Autodesk Inventor part; units mm, degrees
ref_plane "Work Plane1" through (-12, 0, -50) normal (0, -1, 0) x (1, 0, 0)
ref_plane "YZ Plane" through (0, 0, 0) normal (1, 0, 0) x (0, 1, 0)
ref_plane "XZ Plane" through (0, 0, 0) normal (0, 1, 0) x (-1, 0, 0)
sketch "Sketch1" plane through (0, 0, 0) normal (0, 1, 0) x (-1, 0, 0)
  line L0 (12, 50) -> (-12, 50)
  line L1 (-12, 50) -> (-12, -50)
  line L2 (-12, -50) -> (12, -50)
  line L3 (12, -50) -> (12, 50)
  line L4 (12, 50) -> (-12, -50) construction
  line L5 (-12, 50) -> (12, -50) construction
  point P0 (0, 0)
  dimension "d0" = 24
  dimension "d1" = 100
  dimension "d135" = 50
extrude "Extrusion1" add sketch "Sketch1" along normal blind 5
sketch "Sketch3" plane through (0, 5, 0) normal (0, 1, 0) x (1, 0, 0)
  line L0 (-0.2475, -27) -> (0.2525, -27)
  line L1 (0.2525, -27) -> (0.2525, -49)
  line L2 (0.2525, -49) -> (-0.2475, -49)
  line L3 (-0.2475, -49) -> (-0.2475, -27)
  line L4 (12, -50) -> (12, 50)
  line L5 (-12, 50) -> (-12, -50)
  line L6 (-12, -50) -> (12, -50)
  point P0 (0, 0)
  dimension "d24" = 0.5
  dimension "d25" = 11.7475
  dimension "d26" = 22
  dimension "d97" = 11.7525
  dimension "d113" = 1
extrude "Extrusion3" add sketch "Sketch3" along normal blind 30
sketch "Sketch4" plane through (0, 5, 0) normal (0, 1, 0) x (1, 0, 0)
  line L0 (-9.1, -27) -> (9.1, -27)
  line L1 (9.1, -27) -> (9.1, -28)
  line L2 (9.1, -28) -> (-9.1, -28)
  line L3 (-9.1, -28) -> (-9.1, -27)
  line L4 (12, -50) -> (12, 50)
  line L5 (-12, 50) -> (-12, -50)
  line L6 (-12, -50) -> (12, -50)
  point P0 (0, 0)
  dimension "d29" = 1
  dimension "d30" = 2.9
  dimension "d31" = 2.9
  dimension "d114" = 22
extrude "Extrusion4" add sketch "Sketch4" along normal blind 30
sketch "Sketch7" plane through (0, 5, 0) normal (0, 1, 0) x (1, 0, 0)
  line L0 (9.1, -27) -> (8.1, -27)
  line L1 (8.1, -27) -> (8.1, -49)
  line L2 (8.1, -49) -> (9.1, -49)
  line L3 (9.1, -49) -> (9.1, -27)
  line L4 (12, -50) -> (12, 50)
  point P0 (0, 0)
  dimension "d46" = 22
  dimension "d47" = 2.9
  dimension "d48" = 1
extrude "Extrusion7" add sketch "Sketch7" along normal blind 30
sketch "Sketch8" plane through (0, 5, 0) normal (0, 1, 0) x (1, 0, 0)
  line L0 (-9.1, -28) -> (-8.1, -28)
  line L1 (-8.1, -28) -> (-8.1, -49)
  line L2 (-8.1, -49) -> (-9.1, -49)
  line L3 (-9.1, -49) -> (-9.1, -28)
  line L4 (-12, 50) -> (-12, -50)
  point P0 (0, 0)
  dimension "d51" = 21
  dimension "d52" = 2.9
  dimension "d53" = 1
extrude "Extrusion8" add sketch "Sketch8" along normal blind 30
sketch "Sketch9" plane through (0, 5, 0) normal (0, 1, 0) x (1, 0, 0)
  line L0 (-8.3501, -48) -> (-0.2475, -48)
  line L1 (-0.2475, -48) -> (-0.2475, -49)
  line L2 (-0.2475, -49) -> (-8.3501, -49)
  line L3 (-8.3501, -49) -> (-8.3501, -48)
  line L4 (-0.2475, -49) -> (-0.2475, -27)
  line L5 (-12, -50) -> (12, -50)
  point P0 (0, 0)
  point P1 (-0.2475, -28)
  dimension "d56" = 8.1026
  dimension "d57" = 1
  dimension "d58" = 0
  dimension "d59" = 1
extrude "Extrusion9" add sketch "Sketch9" along normal blind 30
sketch "Sketch10" plane through (0, 5, 0) normal (0, 1, 0) x (1, 0, 0)
  line L0 (0.2525, -48) -> (8.3551, -48)
  line L1 (8.3551, -48) -> (8.3551, -49)
  line L2 (8.3551, -49) -> (0.2525, -49)
  line L3 (0.2525, -49) -> (0.2525, -48)
  line L4 (-12, -50) -> (12, -50)
  line L5 (0.2525, -27) -> (0.2525, -49)
  point P0 (0, 0)
  point P1 (0.2525, -28)
  dimension "d62" = 8.1026
  dimension "d63" = 1
  dimension "d64" = 1
  dimension "d65" = 0
extrude "Extrusion10" add sketch "Sketch10" along normal blind 30
sketch "Sketch11" plane through (0, 5, 0) normal (0, 1, 0) x (1, 0, 0)
  point P0 (0, 0)
sketch "Sketch12" plane through (0, 0, 0) normal (0, -1, 0) x (1, 0, 0)
  circle A0 centre (4.5, 43) radius 3.25
  line L0 (12, 50) -> (12, -50)
  circle A1 centre (-4.5, 43) radius 3.25
  line L1 (-12, -50) -> (-12, 50)
  line L2 (-12, 50) -> (12, 50)
  point P0 (0, 0)
  dimension "d69" = 6.5
  dimension "d70" = 7.5
  dimension "d72" = 6.5
  dimension "d73" = 7.5
  dimension "d74" = 7
  dimension "d75" = 7
extrude "Extrusion11" add sketch "Sketch12" along normal blind 20
sketch "Sketch15" plane through (4.5, -20, 43) normal (0, -1, 0) x (1, 0, 0)
  point P0 (-4.5, -43)
extrude "Extrusion12" [suppressed]
sketch "Sketch16" plane through (-4.5, -20, 43) normal (0, -1, 0) x (1, 0, 0)
  point P0 (4.5, -43)
extrude "Extrusion13" [suppressed]
ref_plane "Work Plane1" through (-12, 0, -50) normal (0, -1, 0) x (1, 0, 0)
split body "Split1" result two bodies by plane through (-12, 0, -50) normal (0, -1, 0) first body at (7.2144, -13.3333, 42.5589) (-1.7856, -13.3333, 42.5589)
split "Split2" plane through (-12, 0, -50) removes the side toward (0, -1, 0)
sketch "Sketch20" plane through (0, 0, 0) normal (0, -1, 0) x (1, 0, 0)
  line L0 (-1, 28) -> (-2, 28)
  line L1 (-2, 28) -> (-2, 48)
  line L2 (-2, 48) -> (-1, 48)
  line L3 (-1, 48) -> (-1, 28)
  line L4 (1, 28) -> (2, 28)
  line L5 (2, 28) -> (2, 48)
  line L6 (2, 48) -> (1, 48)
  line L7 (1, 48) -> (1, 28)
  line L8 (-12, -50) -> (-12, 50)
  line L9 (12, 50) -> (12, -50)
  line L10 (-12, 50) -> (12, 50)
  point P0 (0, 0)
  dimension "d84" = 11
  dimension "d85" = 11
  dimension "d86" = 1
  dimension "d87" = 1
  dimension "d88" = 20
  dimension "d89" = 2
extrude "Extrusion14" cut sketch "Sketch20" against normal blind 25.4 bodies 3
sketch "Sketch25" plane through (0, 0, 0) normal (0, -1, 0) x (1, 0, 0)
  circle A0 centre (0, 10) radius 6
  line L0 (12, -50) -> (-12, -50)
  point P0 (0, 0)
  dimension "d109" = 12
  dimension "d110" = 60
extrude "Extrusion18" cut sketch "Sketch25" against normal blind 25.4 bodies 3
sketch "Sketch26" plane through (0, 5, 0) normal (0, 1, 0) x (1, 0, 0)
  point P0 (0, 0)
sketch "Sketch27" plane through (-1, 0, 48) normal (0, 0, -1) x (-1, 0, 0)
  point P0 (-1, 0)
sketch "Sketch28" plane through (0, 5, 0) normal (0, 1, 0) x (1, 0, 0)
  point P0 (0, 0)
sketch "Sketch29" plane through (0, 0, 0) normal (0, -1, 0) x (1, 0, 0)
  circle A0 centre (-6.5, 38) radius 1.5
  circle A1 centre (6.5, 38) radius 1.5
  line L0 (-12, 50) -> (12, 50)
  line L1 (-12, -50) -> (-12, 50)
  line L2 (12, 50) -> (12, -50)
  point P0 (0, 0)
  dimension "d121" = 3
  dimension "d122" = 3
  dimension "d123" = 12
  dimension "d124" = 12
  dimension "d125" = 5.5
  dimension "d126" = 5.5
extrude "Extrusion19" cut sketch "Sketch29" against normal blind 25.4 bodies 3
sketch "Sketch30" plane through (0, 35, 0) normal (0, 1, 0) x (1, 0, 0)
  point P0 (0, 0)
sketch "Sketch31" plane through (0, 5, 0) normal (0, 1, 0) x (1, 0, 0)
  line L0 (-1, -28) -> (1, -28)
  line L1 (1, -28) -> (1, -48)
  line L2 (1, -48) -> (-1, -48)
  line L3 (-1, -48) -> (-1, -28)
  line L4 (-0.2475, -28) -> (-1, -28)
  line L5 (-1, -28) -> (-1, -48)
  line L6 (1, -48) -> (1, -28)
  line L7 (0.2525, -48) -> (1, -48)
  point P0 (0, 0)
  dimension "d129" = 0
  dimension "d130" = 0
  dimension "d131" = 0
  dimension "d132" = 0
extrude "Extrusion20" add sketch "Sketch31" along normal blind 30 bodies 3
sketch "Sketch32" plane through (0, 0, 0) normal (0, -1, 0) x (1, 0, 0)
  point P0 (0, 0)
sketch "Sketch33" plane through (0, 0, 0) normal (0, -1, 0) x (1, 0, 0)
  point P0 (0, 0)
sketch "Sketch34" plane through (0, 0, 0) normal (0, -1, 0) x (1, 0, 0)
  point P0 (0, 0)
sketch "Sketch35" plane through (0, 5, 0) normal (0, 1, 0) x (1, 0, 0)
  point P0 (0, 0)
sketch "Sketch36" plane through (0, 5, 0) normal (0, 1, 0) x (1, 0, 0)
  point P0 (0, 0)
sketch "Sketch37" plane through (0, 5, 0) normal (0, 1, 0) x (1, 0, 0)
  point P0 (0, 0)
sketch "Sketch38" plane through (0, 5, 0) normal (0, 1, 0) x (1, 0, 0)
  point P0 (0, 0)
sketch "Sketch39" plane through (0, 5, 0) normal (0, 1, 0) x (1, 0, 0)
  point P0 (0, 0)
sketch "Sketch40" plane through (0, 5, 0) normal (0, 1, 0) x (1, 0, 0)
  line L0 (2, -28) -> (3, -28)
  line L1 (3, -28) -> (3, -48)
  line L2 (3, -48) -> (2, -48)
  line L3 (2, -48) -> (2, -28)
  line L4 (2, -48) -> (8.1, -48)
  line L5 (8.1, -28) -> (2, -28)
  point P0 (0, 0)
  dimension "d136" = 0
  dimension "d137" = 0
  dimension "d138" = 1
  dimension "d139" = 0
extrude "Extrusion21" add sketch "Sketch40" along normal blind 30 bodies 3
sketch "Sketch41" plane through (0, 5, 0) normal (0, 1, 0) x (1, 0, 0)
  line L0 (-2, -28) -> (-3, -28)
  line L1 (-3, -28) -> (-3, -48)
  line L2 (-3, -48) -> (-2, -48)
  line L3 (-2, -48) -> (-2, -28)
  line L4 (-2, -28) -> (-8.1, -28)
  line L5 (-2, -48) -> (-2, -28)
  line L6 (-8.1, -48) -> (-2, -48)
  point P0 (0, 0)
  dimension "d142" = 0
  dimension "d143" = 0
  dimension "d144" = 0
  dimension "d145" = 1
extrude "Extrusion22" add sketch "Sketch41" along normal blind 30 bodies 3
sketch "Sketch42" plane through (0, 35, 0) normal (0, 1, 0) x (1, 0, 0)
  point P0 (0, 0)
sketch "Sketch43" plane through (0, 35, 0) normal (0, 1, 0) x (1, 0, 0)
  line L0 (9.1, -27) -> (-9.1, -27)
  line L1 (-9.1, -49) -> (9.1, -49)
  line L2 (-0.5, -27) -> (0.5, -27)
  line L3 (0.5, -27) -> (0.5, -49)
  line L4 (0.5, -49) -> (-0.5, -49)
  line L5 (-0.5, -49) -> (-0.5, -27)
  line L6 (1, -48) -> (1, -28)
  point P0 (0, 0)
  dimension "d148" = 1
  dimension "d149" = 0.5
extrude "baffle" add sketch "Sketch43" along normal blind 6 bodies 3
sketch "Sketch45" plane through (0, 0, 0) normal (0, -1, 0) x (1, 0, 0)
  circle A0 centre (-6.5, 38) radius 2.5
  circle A1 centre (-6.5, 38) radius 1.5
  circle A2 centre (-6.5, 38) radius 3.7
  line L0 (-12, 50) -> (12, 50)
  line L1 (0, 50) -> (0, 16)
  circle A3 centre (0, 10) radius 6
  circle A4 centre (6.5, 38) radius 2.5
  circle A5 centre (6.5, 38) radius 3.7
  point P0 (0, 0)
  dimension "d155" = 5
  dimension "d156" = 1.2
extrude "Extrusion25" add sketch "Sketch45" along normal blind 10 contours A2 | A5 bodies 3
sketch "Sketch46" plane through (0, 5, 0) normal (0, 1, 0) x (1, 0, 0)
  line L0 (12, 50) -> (-12, 50)
  line L1 (12, -50) -> (12, 50)
  line L2 (-12, 50) -> (12, 50)
  line L3 (12, 50) -> (12, -2.4141)
  line L4 (12, -2.4141) -> (-12, -2.4141)
  line L5 (-12, -2.4141) -> (-12, 50)
  point P0 (0, 0)
extrude "Extrusion26" cut sketch "Sketch46" against normal through all bodies 3
properties part number "jtd_lid4_20160910"
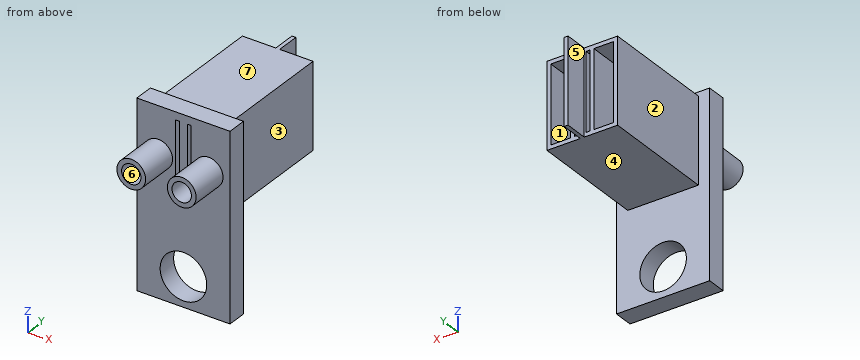
The model under review builds one solid part; all positions refer to its coordinate system, in mm. Face numbers are marked on the shaded views. A direction names the side the tool comes from. Give positions to 0.01 mm unless a question says otherwise; leave off trailing zeros. Write each loop counter-clockwise with the first axis right and the second up, starting at its lowest first coordinate (ties: lowest second). Pieces come first, ordered by that corner, then holes. Notation, with made-up numbers: M 24.25,18 L 78.25,18 A25 ccw 78.25,37 Z; hole C 17.25,28 d9. An arc over 180 degrees is marked long. Write item = value, one per line. Start each with the question number.
Q1. Machinability: for the marked faces 4, 5, 6 and 7, which of the approach directions +Z, -Z, +X, -X, +Y, -Y give a long, thin tool a straight path to every point of the face, cutting with its end or side? Answer none if there is none.
Q2. We need section B-B (y = 14.5). State the section outline as (x, z) points.
Q3. Clearance check with flat-ended pins moving along their axes: pin 1 (0.8 mm diameter, centred on x = 1.5, y = 23, fed in from +Z); pin 2 (1 mm diameter, centred on x = -6, y = 16.5, fed in from -Z); pin 3 (11 mm diameter, centred on y = 25, z = 43, fed in from +X). State where each tip first meets the part, or that it passes through.
Q4. Mouldability with a two-part tool opening along X and no side actions: class the marked faces 1, 2 and 3 as released by +X, released by -X, zero draft, split by the parting line, or undercut.
Q5. For line 1 (X direction, y = 24.5, z = 37.5); line 2 (Z direction, x = 6.5, y = 2.9); line 3 (Z direction, x = 0, y = 2.3), list the stretches that pass through material, from the lowest coordinate up.
Q6. We need section D-D (y = 3). State the section outline as (x, z) points, plus the area to 3 significant figures.
Q7. We need section C-C (z = 33.5). State the section outline as (x, y) points.
Q8. We need section A-A (z = 10). State the section outline as (x, y) points.
Result set:
q1.face_4 = -Z, +X, -X, +Y
q1.face_5 = +Z, -Z, -X, +Y
q1.face_6 = -Y
q1.face_7 = +Z, +X, -X, +Y
q2.outline = M -9.1,27 L 9.1,27 L 9.1,49 L -9.1,49 Z; hole M -8.1,28 L -3,28 L -3,48 L -8.1,48 Z; hole M -2,28 L -1,28 L -1,48 L -2,48 Z; hole M 1,28 L 2,28 L 2,48 L 1,48 Z; hole M 3,28 L 8.1,28 L 8.1,48 L 3,48 Z
q3.pin_1 = 49
q3.pin_2 = 27
q3.pin_3 = 9.1
q4.face_1 = undercut
q4.face_2 = released by -X
q4.face_3 = released by +X
q5.line_1 = -9.1 to -8.1, -3 to -2, -1 to 1, 2 to 3, 8.1 to 9.1
q5.line_2 = 2.41 to 36.5, 39.5 to 50
q5.line_3 = 2.41 to 4, 16 to 50
q6.outline = M -12,2.41 L 12,2.41 L 12,50 L -12,50 Z; hole C -6.5,38 d3; hole C 0,10 d12; hole M -2,28 L -1,28 L -1,48 L -2,48 Z; hole M 1,28 L 2,28 L 2,48 L 1,48 Z; hole C 6.5,38 d3
q6.area = 975 mm2
q7.outline = M -12,0 L -2,0 L -2,35 L -3,35 L -3,5 L -8.1,5 L -8.1,35 L -9.1,35 L -9.1,5 L -12,5 Z; M -1,0 L 1,0 L 1,35 L 0.5,35 L 0.5,41 L -0.5,41 L -0.5,35 L -1,35 Z; M 2,0 L 12,0 L 12,5 L 9.1,5 L 9.1,35 L 8.1,35 L 8.1,5 L 3,5 L 3,35 L 2,35 Z
q8.outline = M -12,0 L -6,0 L -6,5 L -12,5 Z; M 6,0 L 12,0 L 12,5 L 6,5 Z
